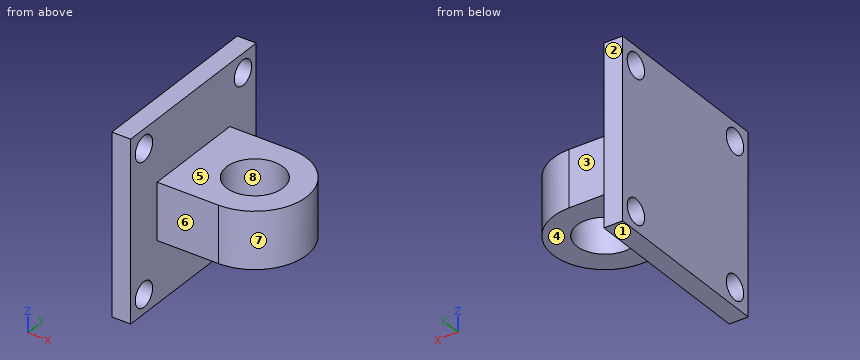
```python
from build123d import *

# Parameters (mm, degrees)
SKETCH1_W           = 241.3
SKETCH1_H           = 241.3
BOSS_EXTRUDE1_DEPTH = 25.4
BOSS_EXTRUDE2_DEPTH = 76.2
HOLE1_D             = 76.2
HOLE1_DEPTH         = 158.75
HOLE2_D             = 33.3502
HOLE2_DEPTH         = 177.8


with BuildPart() as part:
    # Sketch1 → Boss-Extrude1 (new body)
    with BuildSketch(Plane(origin=(25.4, 0, 0), x_dir=(0, 0, -1), z_dir=(1, 0, 0))):
        Rectangle(SKETCH1_W, SKETCH1_H)
    extrude(amount=-BOSS_EXTRUDE1_DEPTH)

    # Sketch2 → Boss-Extrude2 (add)
    with BuildSketch(Plane.XY.offset(38.1)):
        with BuildLine():
            Line((25.4, 69.85), (25.4, -69.85))
            Line((25.4, -69.85), (107.95, -69.85))
            ThreePointArc((107.95, -69.85), (177.8, 0), (107.95, 69.85))
            Line((107.95, 69.85), (25.4, 69.85))
        make_face()
    extrude(amount=-BOSS_EXTRUDE2_DEPTH)

    # Hole1
    with Locations(Plane(origin=(0, 0, -38.1), x_dir=(-1, 0, 0), z_dir=(0, 0, -1))):
        with Locations((-107.95, 0)):
            Hole(HOLE1_D / 2, depth=HOLE1_DEPTH)

    # Hole2
    with Locations(Plane.ZY):
        with Locations((-95.25, -95.25), (-95.25, 95.25), (95.25, -95.25), (95.25, 95.25)):
            Hole(HOLE2_D / 2, depth=HOLE2_DEPTH)


solid = part.part
```
For this review, take the finished solid that the model builds, in its own axes (mm). Face numbers are marked on the shaded views. A direction names the side the tool comes from. Give positions to 0.01 mm unless a question says otherwise; leave off trailing zeros. Order: outer loops, then holes, each group sorted by start corner. A loop starts at its lowest first (then second) coordinate and runs counter-clockwise, first axis right, second up.
1) For the marked faces 1, 2, 3, 4 and 5, list the 3-axis set-ups (+Z, -Z, +X, -X, +Y, -Y) from which the entire face can be reached by the end or side of a thin tool; tool diameter is ignored.
2) Take a section at B-B (x = 12). Give the boundary of the cut face in (y, z), then the cut area to 3 significant figures.
3) Take a section at A-A (z = -95.25). Give the boundary of the cut face in (x, y), then the cut area to 3 significant figures.
4) Wall thickness on line 1 (Z direction, x = 5, y = 95); line 2 (Y direction, x = 12.5, z = 95.25); line 3 (Z direction, x = 18.5, y = 86.5): over which ranges is each line inside the solid? List them lowest first.
5) Insertion check: pin 1 (4 mm diameter, centred on y = 3.5, z = -42, fed in from +X); pin 2 (8 mm diameter, centred on y = -75, z = -9.5, fed in from -X); pin 3 (5 mm diameter, centred on x = 129, z = 20.5, fed in from +Y); pin 4 (4 mm diameter, centred on x = 142, y = 29, fed in from -Z). Each pin has a flat end and moves straight along its axis. Give the tip position at first contact, or say it passes through.
6) The part is to be moulded in two halves that separate along Y. For the marked faces 6, 7 and 8, say which applies: released by +Y, released by -Y, zero draft, split by the parting line, or undercut.
7) Take a section at D-D (y = 4). Give the boundary of the cut face in (x, z), then the cut area to 3 significant figures.
Derived:
1. face 1: -Z, +X, -X, +Y, -Y
1. face 2: +Z, -Z, +X, -X, +Y
1. face 3: +Z, -Z, +X, +Y
1. face 4: -Z, +X, +Y, -Y
1. face 5: +Z, +X, +Y, -Y
2. outline: (-120.65, -120.65) - (120.65, -120.65) - (120.65, 120.65) - (-120.65, 120.65) - close; hole circle Ø33.35 at (-95.25, -95.25); hole circle Ø33.35 at (-95.25, 95.25); hole circle Ø33.35 at (95.25, -95.25); hole circle Ø33.35 at (95.25, 95.25)
2. area: 54,700 mm2
3. outline: (0, -120.65) - (25.4, -120.65) - (25.4, -111.93) - (0, -111.93) - close; (0, -78.57) - (25.4, -78.57) - (25.4, 78.57) - (0, 78.57) - close; (0, 111.93) - (25.4, 111.93) - (25.4, 120.65) - (0, 120.65) - close
3. area: 4,430 mm2
4. line 1: z = -120.65 to -111.92, -78.58 to 78.58, 111.92 to 120.65
4. line 2: y = -120.65 to -111.93, -78.57 to 78.57, 111.93 to 120.65
4. line 3: z = -120.65 to -109.44, -81.06 to 81.06, 109.44 to 120.65
5. pin 1: stops at x = 25.4
5. pin 2: stops at x = 0
5. pin 3: stops at y = 67.34
5. pin 4: stops at z = -38.1
6. face 6: released by -Y
6. face 7: split by the parting line
6. face 8: undercut
7. outline: (0, -120.65) - (25.4, -120.65) - (25.4, -38.1) - (70.06, -38.1) - (70.06, 38.1) - (25.4, 38.1) - (25.4, 120.65) - (0, 120.65) - close; (145.84, -38.1) - (177.69, -38.1) - (177.69, 38.1) - (145.84, 38.1) - close
7. area: 12,000 mm2
